Can you work these out from the model? Positions are in its coordinate system, mm. Coordinates: 2 decimals unless noted, no trailing zeros. Loops run counter-clockwise (first coordinate to the right, second up) from the corner with the lowest first, then second, coordinate; pieces in that order, holes last. Notation, with made-up numbers: (37.5, 25.25) - (45.5, 25.25) arc R32 ccw to (45.5, 63.25) - close; hole circle Ø3 at (6, 52.25). An arc over 180 degrees is marked (long way). Put each result on its own line as item: value. Start each with the question number.
from build123d import *

# Parameters (mm, degrees)
F1_DEPTH = 1090


with BuildPart() as f1:
    # F0 (on Front) → F1 (new body)
    with BuildSketch(Plane.XZ):
        with BuildLine():
            Line((-29.841657, 19.006058), (-29.956796, 0))
            Line((-29.956796, 0), (10.043204, 0))
            Line((10.043204, 0), (10.043204, 19))
            ThreePointArc((10.043204, 19), (9.750311, 19.707107), (9.043204, 20))
            Line((9.043204, 20), (7.918096, 20))
            ThreePointArc((7.918096, 20), (6.550256, 19.459114), (5.922262, 18.129013))
            Line((5.922262, 18.129013), (5.315472, 8.741974))
            ThreePointArc((5.315472, 8.741974), (4.059483, 6.081772), (1.323803, 5))
            Line((1.323803, 5), (-21.161531, 5))
            ThreePointArc((-21.161531, 5), (-23.903058, 6.087264), (-25.154203, 8.757985))
            Line((-25.154203, 8.757985), (-25.721741, 18.121007))
            ThreePointArc((-25.721741, 18.121007), (-26.347313, 19.456368), (-27.718077, 20))
            Line((-27.718077, 20), (-28.841675, 20))
            ThreePointArc((-28.841675, 20), (-29.546637, 19.709245), (-29.841657, 19.006058))
        make_face()
    extrude(amount=F1_DEPTH)


solid = f1.part
Q1. Please list where these lines run through material, in increasing order: line 1 along X through (y, z) = (-241, 8); line 2 along X through (y, z) = (-334, 8.5); line 3 along Z through (x, y) = (-16.5, -677). Write a range as [from, to].
Q2. I want a section at B-B on y = -527.5. List the corners of the cut face in (x, z) for me.
Q3. We'd pull the mould along X, two halves only. Please class faces 1 (the flat face through (10.043, -537, 9)), 2 (the flat face through (-10, -537, 0)), 3 (the flat face through (-10, -537, 5)): released by +X, released by -X, zero draft, split by the parting line, or undercut.
Q4. I want a section at A-A on z = 12. List the corners of the cut face in (x, y) for me, and give its area (3 significant figures).
Q5. I want a section at C-C on x = -8. List the corners of the cut face in (y, z) for me, and give its area (3 significant figures).
Q6. Will these pins go through, and if not, where does the flat tip stop? pin 1 (1.5 mm diameter, centred on y = -648, z = 4.5, fed in from -X); pin 2 (6.5 mm diameter, centred on x = -15, y = -549.5, fed in from +Z).
Calculated:
1. line 1: [-29.91, -25.03], [5.2, 10.04]
1. line 2: [-29.91, -25.13], [5.29, 10.04]
1. line 3: [0, 5]
2. outline: (-29.96, 0) - (10.04, 0) - (10.04, 19) arc R1 ccw to (9.04, 20) - (7.92, 20) arc R2 ccw to (5.92, 18.13) - (5.32, 8.74) arc R4 cw to (1.32, 5) - (-21.16, 5) arc R4 cw to (-25.15, 8.76) - (-25.72, 18.12) arc R2 ccw to (-27.72, 20) - (-28.84, 20) arc R1 ccw to (-29.84, 19.01) - close
3. face 1: released by +X
3. face 2: zero draft
3. face 3: undercut
4. outline: (-29.88, -1090) - (-25.35, -1090) - (-25.35, 0) - (-29.88, 0) - close; (5.53, -1090) - (10.04, -1090) - (10.04, 0) - (5.53, 0) - close
4. area: 9,870 mm2
5. outline: (-1090, 0) - (0, 0) - (0, 5) - (-1090, 5) - close
5. area: 5,450 mm2
6. pin 1: x = -29.93
6. pin 2: z = 5
